from build123d import *

# Parameters (mm, degrees)
F0_W     = 63.920457
F0_H     = 36.818182
F0_R     = 12.305973
F1_DEPTH = 6.3
F2_W     = 63.664775
F2_H     = 6.90341
F3_DEPTH = 58.4


with BuildPart() as f1:
    # F0 (on Top) → F1 (new body)
    with BuildSketch(Plane.XY):
        with Locations((-0.127842, 1.150568)):
            Rectangle(F0_W, F0_H)
        Circle(F0_R, mode=Mode.SUBTRACT)
    extrude(amount=F1_DEPTH)

    # F2 (on face) → F3 (join)
    with BuildSketch(Plane(origin=(0, 0, 0), x_dir=(1, 0, 0), z_dir=(0, 0, -1))):
        with Locations((-0.255683, 20.710228)):
            Rectangle(F2_W, F2_H)
    extrude(amount=-F3_DEPTH)


solid = f1.part
Source: CAD feature listing. Evaluate the final solid. Frame: model axes, mm. A direction names the side the tool comes from. Coordinates: 2 decimals unless noted, no trailing zeros. Order: outer loops, then holes, each group sorted by start corner. A loop starts at its lowest first (then second) coordinate and runs counter-clockwise, first axis right, second up. Notation, with made-up numbers: M 36.25,12 L 45.25,12 A16 cw 45.25,32 Z; hole C 47.25,33 d5. An arc over 180 degrees is marked long. Write each question's results on one line, items separated by ' | '. Start each with the question number.
1. Reachability of faces 4 (the face through (-1, -21, 58.4)), 5 (the face through (-1, 14, 6.3)) from +Z, -Z, +X, -X, +Y, -Y: full face, straight path, thin tool, end or side. Return the list, or none.
2. Section A-A, the plane x = 0. Return the cut outline in (y, z), then the cut area to 3 significant figures.
3. Pin query (flat end, axial travel): pin 1 (2 mm diameter, centred on x = 23.5, y = 11.5, fed in from -Z); pin 2 (11 mm diameter, centred on x = 12, y = 10, fed in from +Z); pin 3 (5.5 mm diameter, centred on y = -21, z = 23, fed in from +X); pin 4 (4 mm diameter, centred on x = -8.5, z = 34, fed in from +Y). Return the tip coordinate at first contact, or that it passes through.
4. Section C-C, the plane x = -21. Return the cut outline in (y, z), then the cut area to 3 significant figures.
5. Material intervals for L1, parallel to Y at x = 0, z = 3.5; L2, parallel to Y at x = -20, z = 42; L3, parallel to Z at x = 20.5, y = -12, sorted ascending.
6. Draft query along Y for faces 1 (the face through (-1, 19.56, 3)), 2 (the face through (-1.6, 12.2, 3.1)), 3 (the face through (31.577, -21, 29)). Return one class per face: +Y half, -Y half, draft (parallel to the pull), parting line (faces both ways), or undercut.
7. Section D-D, the plane y = 13.5. Return the cut outline in (x, z).
8. Section B-B, the plane y = 0. Return the cut outline in (x, z), then the cut area to 3 significant figures.
Solution:
1) face 4: +Z, +X, -X, +Y, -Y | face 5: +Z, +X, -X, +Y
2) outline: M -24.16,0 L -12.31,0 L -12.31,6.3 L -17.26,6.3 L -17.26,58.4 L -24.16,58.4 Z; M 12.31,0 L 19.56,0 L 19.56,6.3 L 12.31,6.3 Z | area: 480 mm²
3) pin 1: z = 0 | pin 2: z = 6.3 | pin 3: x = 31.58 | pin 4: y = -17.26
4) outline: M -24.16,0 L 19.56,0 L 19.56,6.3 L -17.26,6.3 L -17.26,58.4 L -24.16,58.4 Z | area: 635 mm²
5) L1: -24.16 to -12.31, 12.31 to 19.56 | L2: -24.16 to -17.26 | L3: 0 to 6.3
6) face 1: +Y half | face 2: undercut | face 3: draft
7) outline: M -32.09,0 L 31.83,0 L 31.83,6.3 L -32.09,6.3 Z
8) outline: M -32.09,0 L -12.31,0 L -12.31,6.3 L -32.09,6.3 Z; M 12.31,0 L 31.83,0 L 31.83,6.3 L 12.31,6.3 Z | area: 248 mm²
